Input: part model. Units: mm. Frame: model coordinates. Give positions to 0.01 mm unless a question says otherwise; leave off trailing zeros. Write each loop counter-clockwise with the first axis right and the second up, starting at its lowest first coordinate (ties: lowest second). Pieces come first, ordered by that corner, then holes. Notation, with made-up numbers: M -20.5,-23.5 L 27.5,-23.5 A20 cw 27.5,-18.5 Z; hole C -20,10.5 d9. An arc over 180 degrees is marked long. Use CSV: the item, a comma, the result in double quotes. Start each with the question number.
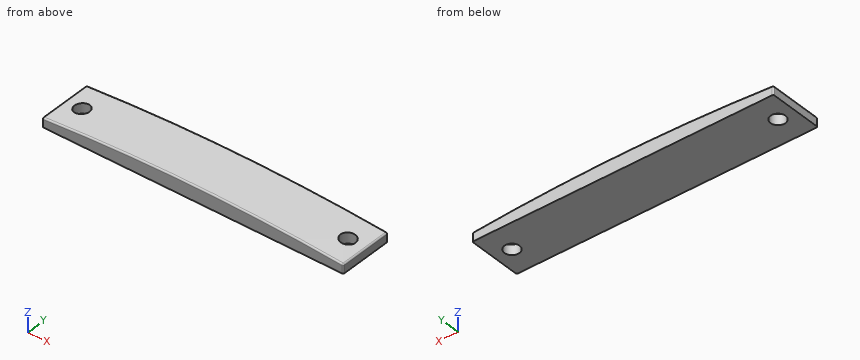
from build123d import *

# Parameters (mm, degrees)
F1_DEPTH      = 18
F1_DEPTH_BACK = 18
F2_R          = 5
F3_DEPTH      = 25
F4_R          = 1


with BuildPart() as f1:
    # F0 (on Front) → F1 (new body, two sides)
    with BuildSketch(Plane.XZ) as f1_sk:
        with BuildLine():
            Line((-100, 6), (-100, 0))
            Line((-100, 0), (100, 0))
            Line((100, 0), (100, 6))
            ThreePointArc((100, 6), (0, 10), (-100, 6))
        make_face()
    extrude(amount=F1_DEPTH)
    extrude(f1_sk.sketch, amount=-F1_DEPTH_BACK)

    # F2 (on Top) → F3 (cut)
    with BuildSketch(Plane.XY):
        with Locations((-88.35, 0)):
            Circle(F2_R)
        with Locations((88.35, 0)):
            Circle(F2_R)
    extrude(amount=F3_DEPTH, mode=Mode.SUBTRACT)

    # F4
    f4_edges = [f1.edges().sort_by_distance(p)[0] for p in [
        (-100, 0, 6),
        (0, -18, 10),
        (100, 0, 6),
        (0, 18, 10),
        (100, -18, 3),
        (100, 18, 3),
        (-100, 18, 3),
        (-100, -18, 3),
    ]]
    fillet(f4_edges, radius=F4_R)


solid = f1.part
Q1. Section B-B, the plane y = 12.5. Return the cut outline in (x, z).
Q2. First-contact query: pin 1 Ø8 at (x, y) = (-88.35, 0) entering from -Z. Flat tip, straight axial feed; report the tip coordinate or a pass-through.
Q3. Section A-A, the plane y = 0. Return the cut outline in (x, z).
Q4. Material intervals for L1, parallel to X at y = 0, z = 4.75; L2, parallel to Y at x = 88.35, z = 4; L3, parallel to X at y = 0, z = 5.75, sorted ascending. Write a range as [from, to].
Check result:
1,outline,"M -100,0 L 100,0 L 100,5.08 A1 ccw 99.08,6.07 A1252 ccw -99.08,6.07 A1 ccw -100,5.08 Z"
2,pin 1,"passes through"
3,outline,"M -100,0 L -93.35,0 L -93.35,6.52 A1252 ccw -99.08,6.07 A1 ccw -100,5.08 Z; M -83.35,0 L 83.35,0 L 83.35,7.22 A1252 ccw -83.35,7.22 Z; M 93.35,0 L 100,0 L 100,5.08 A1 ccw 99.08,6.07 A1252 ccw 93.35,6.52 Z"
4,L1,"x = [-100, -93.35], [-83.35, 83.35], [93.35, 100]"
4,L2,"y = [-18, -5], [5, 18]"
4,L3,"x = [-99.74, -93.35], [-83.35, 83.35], [93.35, 99.74]"
